For this review, take the finished solid that the model builds, in its own axes (mm). Face numbers are marked on the shaded views. A direction names the side the tool comes from. Give positions to 0.01 mm unless a question says otherwise; leave off trailing zeros. Write each loop counter-clockwise with the first axis right and the second up, starting at its lowest first coordinate (ties: lowest second). Pieces come first, ordered by that corner, then holes.
Q1. Machinability: for the marked faces 4, 5, 6 and 7, which of the approach directions +Z, -Z, +X, -X, +Y, -Y give a long, thin tool a straight path to every point of the face, cutting with its end or side? Answer none if there is none.
Q2. For line 1 (X direction, y = 22, z = 6.25); line 2 (X direction, y = 13, z = 6.25); line 3 (X direction, y = -15, z = -11), list the stretches that pass through material, from the lowest coordinate up.
Q3. Insertion check: P1, Ø8.5, axis at x = -43.14, z = 6.25, coming from the +Y side; P2, Ø14.5, axis at x = 18, z = -11, coming from the +Y side; P3, Ø4, axis at x = -6.5, z = 7.5, coming from the -Y side. Each pin has a flat end and moves straight along its axis. Give the tip position at first contact, or say it passes through.
Q4. We need section B-B (z = -2). Write out the cut boundary in (x, y), then the cut area to 3 significant figures.
Q5. We need section C-C (z = -7.25). Write out the cut boundary in (x, y).
Q6. Mouldability with a two-part tool opening along Z and no side actions: class the marked faces 1, 2 and 3 as released by +Z, released by -Z, zero draft, split by the parting line, or undercut.
Q7. We need section A-A (y = -8.5). Write out the cut boundary in (x, z).
Q8. We need section D-D (y = 22). Write out the cut boundary in (x, z).
```python
from build123d import *

# Parameters (mm, degrees)
BOSS_EXTRUDE1_DEPTH              = 12.5
SKETCH8_W                        = 13
SKETCH8_H                        = 10
BOSS_EXTRUDE2_DEPTH              = 14.5
F_10_0_1935_DIAMETER_HOLE1_D     = 4.9149
SKETCH14_R                       = 3.5
BOSS_EXTRUDE3_DEPTH              = 12.6
SKETCH23_R                       = 0.8
CUT_EXTRUDE3_DEPTH               = 30
SKETCH24_R                       = 0.8
CUT_EXTRUDE4_DEPTH               = 30
F_3_8_0_375_DIAMETER_HOLE5_D     = 9.525
F_3_8_0_375_DIAMETER_HOLE5_DEPTH = 10
F_3_8_0_375_DIAMETER_HOLE5_TIP   = 2.861598698


with BuildPart() as part:
    # Sketch6 → Boss-Extrude1 (new body)
    with BuildSketch(Plane.XY):
        Polygon((-54.693316182, -23.370226934), (-54.693316182, 19.129773066), (-15.093316182, 19.129773066), (-15.093316182, 6.803860506), (-41.693316182, 6.803860506), (-41.693316182, -23.370226934), align=None)
    extrude(amount=BOSS_EXTRUDE1_DEPTH)

    # Sketch8 → Boss-Extrude2 (add)
    with BuildSketch(Plane(origin=(0, 0, 0), x_dir=(-1, 0, 0), z_dir=(0, 0, -1))):
        with Locations((48.193316182, -18.370226934)):
            Rectangle(SKETCH8_W, SKETCH8_H)
    extrude(amount=BOSS_EXTRUDE2_DEPTH)

    # Mirror1: part across plane


with BuildPart() as part_1:
    add(part.part)
    add(part.part.mirror(Plane(origin=(-15.093316182, 6.803860506, 12.5), x_dir=(0, 0, 1), z_dir=(-1, 0, 0))))

    # #10 (0.1935) Diameter Hole1 (through all)
    with Locations(Plane(origin=(0, -13.370226934, 0), x_dir=(1, 0, 0), z_dir=(0, 1, 0))):
        with Locations((-48.193316182, 7.25), (18.006683818, 7.25)):
            Hole(F_10_0_1935_DIAMETER_HOLE1_D / 2)

    # Sketch14 → Boss-Extrude3 (add)
    with BuildSketch(Plane(origin=(0, 19.129773066, 0), x_dir=(1, 0, 0), z_dir=(0, 1, 0))):
        with Locations((-28.093316182, -6.25)):
            Circle(SKETCH14_R)
        with Locations((-2.093316182, -6.25)):
            Circle(SKETCH14_R)
    extrude(amount=BOSS_EXTRUDE3_DEPTH)

    # Sketch23 → Cut-Extrude3 (cut)
    with BuildSketch(Plane(origin=(0, 31.729773066, 0), x_dir=(1, 0, 0), z_dir=(0, 1, 0))):
        with Locations((-2.093316182, -6.25)):
            Circle(SKETCH23_R)
    extrude(amount=-CUT_EXTRUDE3_DEPTH, mode=Mode.SUBTRACT)

    # Sketch24 → Cut-Extrude4 (cut)
    with BuildSketch(Plane(origin=(0, 31.729773066, 0), x_dir=(1, 0, 0), z_dir=(0, 1, 0))):
        with Locations((-28.093316182, -6.25)):
            Circle(SKETCH24_R)
    extrude(amount=-CUT_EXTRUDE4_DEPTH, mode=Mode.SUBTRACT)

    # 3/8 (0.375) Diameter Hole5
    with Locations(Plane(origin=(-43.143316182, 19.129773066, 6.25), x_dir=(0, 0, 1), z_dir=(0, 1, 0))):
        with Locations((0, 0), (0, 56.1)):
            Hole(F_3_8_0_375_DIAMETER_HOLE5_D / 2, depth=F_3_8_0_375_DIAMETER_HOLE5_DEPTH)
            with Locations((0, 0, -(F_3_8_0_375_DIAMETER_HOLE5_DEPTH + F_3_8_0_375_DIAMETER_HOLE5_TIP / 2))):  # 118° drill point
                Cone(0, F_3_8_0_375_DIAMETER_HOLE5_D / 2, F_3_8_0_375_DIAMETER_HOLE5_TIP, mode=Mode.SUBTRACT)


solid = part_1.part
```
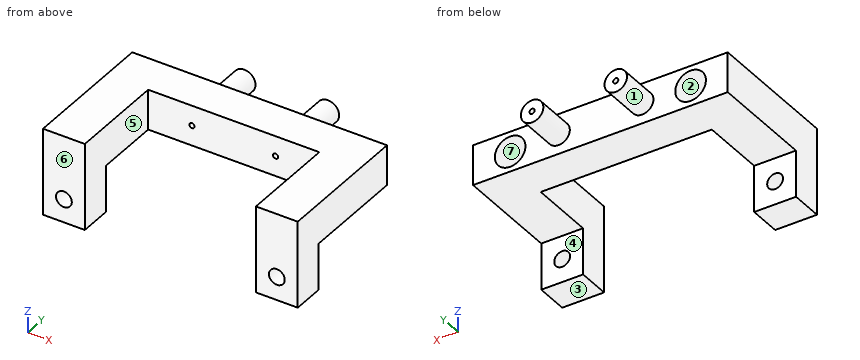
Computed:
1. face 4: -Z, +X, -X, +Y
1. face 5: +Z, -Z, -Y
1. face 6: +Z, -Z, +X, -X, -Y
1. face 7: +Y
2. line 1: x = -31.59 to -28.89, -27.29 to -24.59, -5.59 to -2.89, -1.29 to 1.41
2. line 2: x = -54.69 to -47.91, -38.38 to -28.89, -27.29 to -2.89, -1.29 to 8.19, 17.72 to 24.51
2. line 3: x = -54.69 to -41.69, 11.51 to 24.51
3. P1: stops at y = 8.82
3. P2: stops at y = -13.37
3. P3: stops at y = 6.8
4. outline: (-54.69, -23.37) - (-41.69, -23.37) - (-41.69, -13.37) - (-54.69, -13.37) - close; (11.51, -23.37) - (24.51, -23.37) - (24.51, -13.37) - (11.51, -13.37) - close
4. area: 260 mm2
5. outline: (-54.69, -23.37) - (-50.65, -23.37) - (-50.65, -13.37) - (-54.69, -13.37) - close; (-45.74, -23.37) - (-41.69, -23.37) - (-41.69, -13.37) - (-45.74, -13.37) - close; (11.51, -23.37) - (15.55, -23.37) - (15.55, -13.37) - (11.51, -13.37) - close; (20.46, -23.37) - (24.51, -23.37) - (24.51, -13.37) - (20.46, -13.37) - close
6. face 1: split by the parting line
6. face 2: undercut
6. face 3: released by -Z
7. outline: (-54.69, 0) - (-41.69, 0) - (-41.69, 12.5) - (-54.69, 12.5) - close; (11.51, 0) - (24.51, 0) - (24.51, 12.5) - (11.51, 12.5) - close
8. outline: circle Ø7 at (-28.09, 6.25); circle Ø7 at (-2.09, 6.25); hole circle Ø1.6 at (-28.09, 6.25); hole circle Ø1.6 at (-2.09, 6.25)
